The model under review builds one solid part; all positions refer to its coordinate system, in mm. Face numbers are marked on the shaded views. A direction names the side the tool comes from. Coordinates: 2 decimals unless noted, no trailing zeros. One line per item, written item: value.
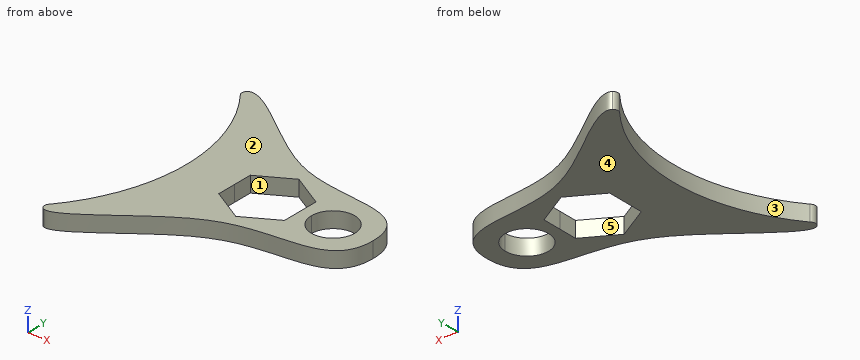
Autodesk Inventor part; units mm, degrees
ref_plane "YZ Plane" through (0, 0, 0) normal (1, 0, 0) x (0, 1, 0)
ref_plane "XZ Plane" through (0, 0, 0) normal (0, 1, 0) x (-1, 0, 0)
ref_plane "XY Plane" through (0, 0, 0) normal (0, 0, 1) x (1, 0, 0)
sketch "Sketch1" plane through (0, 0, 0) normal (0, 0, 1) x (1, 0, 0)
  line L0 (25.3998, 3.6661) -> (28.5748, 1.833)
  line L1 (28.5748, -1.8332) -> (28.5748, 1.833)
  line L2 (28.5748, -1.8332) -> (25.3998, -3.6663)
  line L3 (22.2248, -1.8332) -> (25.3998, -3.6663)
  line L4 (22.2248, -1.8332) -> (22.2248, 1.833)
  line L5 (25.3998, 3.6661) -> (22.2248, 1.833)
  arc A0 (13.9103, 11.4928) -> (13.8254, 10.7824) centre (14.226, 11.0948) ccw
  arc A1 (13.5904, -11.0771) -> (13.7656, -11.9524) centre (13.9159, -11.4671) ccw
  arc A2 (13.5904, -11.0771) -> (13.8254, 10.7824) centre (0, 0) ccw
  circle A3 centre (31.7498, -0.0001) radius 2.0955
  line L6 (31.7498, -0.0001) -> (19.0498, -0.0001)
  line L7 (13.9103, 11.4928) -> (14.9529, 12.3199) construction
  line L8 (14.9529, 12.3199) -> (21.939, 5.9941) construction
  line L9 (21.939, 5.9941) -> (26.2427, 4.1527) construction
  line L10 (26.2427, 4.1527) -> (30.9051, 4.1527) construction
  line L11 (30.9051, 4.1527) -> (35.6157, 3.494) construction
  line L12 (35.6157, 3.494) -> (35.6157, -0.0001) construction
  spline S0 degree 4 poles (13.9103, 11.4928) (14.9529, 12.3199) (21.939, 5.9941) (26.2427, 4.1527) (30.9051, 4.1527) (35.6157, 3.494) (35.6157, -0.0001) knots 1 1 1 1 1 2 3 4 4 4 4 4
  line L13 (13.7656, -11.9524) -> (14.9529, -12.3201) construction
  line L14 (14.9529, -12.3201) -> (21.939, -5.9943) construction
  line L15 (21.939, -5.9943) -> (26.2427, -4.1529) construction
  line L16 (26.2427, -4.1529) -> (30.9051, -4.1529) construction
  line L17 (30.9051, -4.1529) -> (35.6157, -3.4942) construction
  line L18 (35.6157, -3.4942) -> (35.6157, -0.0001) construction
  spline S1 degree 4 poles (13.7656, -11.9524) (14.9529, -12.3201) (21.939, -5.9943) (26.2427, -4.1529) (30.9051, -4.1529) (35.6157, -3.4942) (35.6157, -0.0001) knots 1 1 1 1 1 2 3 4 4 4 4 4
  point P0 (0, 0)
  point P1 (16.4691, 5.9941)
  point P2 (16.469, -5.9943)
  point P3 (25.3998, -0.0001)
  dimension "d31" = 3.6662
  dimension "d32" = 3.6662
  dimension "d34" = 3.6662
  dimension "d35" = 3.6662
  dimension "d36" = 3.6662
  dimension "d37" = 3.6662
  dimension "d44" = 4.191
extrude "Extrusion6" add sketch "Sketch1" along normal blind 1.524
properties part number "gear-interface"
(1) For L1, parallel to Y at x = 16, z = 0.5; L2, parallel to Y at x = 32.75, z = 0.4; L3, parallel to X at y = 7.25, z = 1.15, list the stretches that pass through material, from the lowest coordinate up.
Geometry results:
L1: y = -11.03 to -7.17, 7.17 to 10.94
L2: y = -3.72 to -1.84, 1.84 to 3.72
L3: x = 15.96 to 21.14
(2) Mouldability with a two-part tool opening along X and no side actions: class the marked faces 1, 2 and 3 as +X half, -X half, draft (parallel to the pull), parting line (faces both ways), or undercut.
Geometry results:
face 1: undercut
face 2: draft
face 3: -X half
(3) We need section A-A, the plane z = 0.9. Count the separate pieces of the cut face and the enclosed holes in it, plus the area to 3 significant figures.
Geometry results:
separate pieces: 1
enclosed holes: 2
area: 171 mm2
(4) Tool access review of the marked faces 4 and 5: name each direction out of +Z, -Z, +X, -X, +Y, -Y from which nothing blocks a thin tool from reaching the whole face with its end or side.
Geometry results:
face 4: -Z, +X, -X, +Y, -Y
face 5: +Z, -Z
(5) Insertion check: pin 1 Ø0.5 at (y, z) = (-1.5, 1) entering from -X; pin 2 Ø3 at (x, y) = (27.5, 7.5) entering from +Z. Each pin has a flat end and moves straight along its axis. Give the tip position at first contact, or say it passes through.
Geometry results:
pin 1: stops at x = 17.45
pin 2: passes through
